Can you work these out from the model? Positions are in its coordinate system, mm. Coordinates: 2 decimals unless noted, no trailing zeros. Loops run counter-clockwise (first coordinate to the right, second up) from the corner with the lowest first, then second, coordinate; pieces in that order, holes last.
```python
from build123d import *

# Parameters (mm, degrees)
F0_R     = 4
F1_DEPTH = 8
F3_DEPTH = 4


with BuildPart() as f1:
    # F0 (on Top) → F1 (new body)
    with BuildSketch(Plane.XY):
        Circle(F0_R)
    extrude(amount=F1_DEPTH)

    # F2 (on face) → F3 (cut)
    with BuildSketch(Plane.XY.offset(8)):
        with BuildLine():
            ThreePointArc((3, 0), (2.12132, 2.12132), (0, 3))
            ThreePointArc((0, 3), (-2.12132, 2.12132), (-3, 0))
            ThreePointArc((-3, 0), (-2.12132, -2.12132), (0, -3))
            ThreePointArc((0, -3), (2.12132, -2.12132), (3, 0))
        make_face()
    extrude(amount=-F3_DEPTH, mode=Mode.SUBTRACT)


solid = f1.part
```
Item 1: Suppose I cut it at C-C, the plane z = 0.75. Please give me the cut outline in (x, y).
Results are:
outline: circle Ø8 at (0, 0)
Item 2: Suppose I cut it at B-B, the plane y = -0.5. Please give me the cut outline in (x, z).
Results are:
outline: (-3.97, 0) - (3.97, 0) - (3.97, 8) - (2.96, 8) - (2.96, 4) - (-2.96, 4) - (-2.96, 8) - (-3.97, 8) - close
Item 3: We'd pull the mould along X, two halves only. Please class faces 1 (the face through (-0.867, -3.905, 3.944)), 2 (the face through (1, 3, 8)), 3 (the face through (0, 0, 4)): +X half, -X half, draft (parallel to the pull), parting line (faces both ways), or undercut.
Results are:
face 1: parting line
face 2: draft
face 3: undercut
Item 4: I need wall thicknesses on line 1 along Z through (x, y) = (-1.25, 1.5); line 2 along X through (y, z) = (-0.25, 7.5); line 3 along X through (y, z) = (1, 6). Which ranges of each line are inside material? Lowest first, please.
Results are:
line 1: z = 0 to 4
line 2: x = -3.99 to -2.99, 2.99 to 3.99
line 3: x = -3.87 to -2.83, 2.83 to 3.87
Item 5: Suppose I cut it at A-A, the plane x = 1.25. Please give me the cut outline in (y, z).
Results are:
outline: (-3.8, 0) - (3.8, 0) - (3.8, 8) - (2.73, 8) - (2.73, 4) - (-2.73, 4) - (-2.73, 8) - (-3.8, 8) - close
Item 6: Suppose I cut it at D-D, the plane y = 3.5. Please give me the cut outline in (x, z).
Results are:
outline: (-1.94, 0) - (1.94, 0) - (1.94, 8) - (-1.94, 8) - close
Item 7: I'm going to push flat-ended pins straight in: P1, Ø3, axis at y = 2.5, z = 4, coming from the -X side; P2, Ø2, axis at y = -2.5, z = 4.5, coming from the -X side; P3, Ø2, axis at y = 3, z = 4, coming from the +X side. Where does each tip first touch, or does it pass through?
Results are:
P1: stops at x = -3.87
P2: stops at x = -3.71
P3: stops at x = 3.46
